Model file for the job. Use its own axes, mm. A direction names the side the tool comes from. Coordinates: 2 decimals unless noted, no trailing zeros. Loops run counter-clockwise (first coordinate to the right, second up) from the corner with the lowest first, then second, coordinate; pieces in that order, holes last. Notation, with made-up numbers: (-12.75, 88.5) -> (28.25, 88.5) arc R33 ccw to (28.25, 120.5) -> close; hole circle Ø5 at (75, 76.25). An arc over 180 degrees is marked (long way). Use one line per item in the form item = value.
```python
from build123d import *

# Parameters (mm, degrees)
SKETCH_1_R          = 24.5
SKETCH_1_R_2        = 2.1
EXTRUDE_1_DEPTH     = 2
CUT_EXTRUDE_1_DEPTH = 10


with BuildPart() as part:
    # 草图1 → 凸台-拉伸1 (new body)
    with BuildSketch(Plane.XY):
        with BuildLine():
            Line((-50, 15), (-50, -15))
            ThreePointArc((-50, -15), (-49.077002077, -17.894486839), (-46.648778375, -19.720331542))
            Line((-46.648778375, -19.720331542), (-11.211692948, -32.098254489))
            ThreePointArc((-11.211692948, -32.098254489), (0, -34), (11.211692948, -32.098254489))
            Line((11.211692948, -32.098254489), (46.648778375, -19.720331542))
            ThreePointArc((46.648778375, -19.720331542), (49.077002077, -17.894486839), (50, -15))
            Line((50, -15), (50, 15))
            ThreePointArc((50, 15), (49.077002077, 17.894486839), (46.648778375, 19.720331542))
            Line((46.648778375, 19.720331542), (11.211692948, 32.098254489))
            ThreePointArc((11.211692948, 32.098254489), (0, 34), (-11.211692948, 32.098254489))
            Line((-11.211692948, 32.098254489), (-46.648778375, 19.720331542))
            ThreePointArc((-46.648778375, 19.720331542), (-49.077002077, 17.894486839), (-50, 15))
        make_face()
        Circle(SKETCH_1_R, mode=Mode.SUBTRACT)
        with Locations((0, 29)):
            Circle(SKETCH_1_R_2, mode=Mode.SUBTRACT)
        with Locations((25.11473671, 14.5)):
            Circle(SKETCH_1_R_2, mode=Mode.SUBTRACT)
        with Locations((25.11473671, -14.5)):
            Circle(SKETCH_1_R_2, mode=Mode.SUBTRACT)
        with Locations((0, -29)):
            Circle(SKETCH_1_R_2, mode=Mode.SUBTRACT)
        with Locations((-25.11473671, -14.5)):
            Circle(SKETCH_1_R_2, mode=Mode.SUBTRACT)
        with Locations((-25.11473671, 14.5)):
            Circle(SKETCH_1_R_2, mode=Mode.SUBTRACT)
        with Locations((-45, 15)):
            Circle(SKETCH_1_R_2, mode=Mode.SUBTRACT)
        with Locations((-45, -15)):
            Circle(SKETCH_1_R_2, mode=Mode.SUBTRACT)
        with Locations((45, -15)):
            Circle(SKETCH_1_R_2, mode=Mode.SUBTRACT)
        with Locations((45, 15)):
            Circle(SKETCH_1_R_2, mode=Mode.SUBTRACT)
    extrude(amount=EXTRUDE_1_DEPTH)

    # 草图2 → 切除-拉伸1 (cut)
    with BuildSketch(Plane.XY.offset(2)):
        with BuildLine():
            Line((-43, 11), (-31, 11))
            ThreePointArc((-31, 11), (-29.585786438, 10.414213562), (-29, 9))
            Line((-29, 9), (-29, -9))
            ThreePointArc((-29, -9), (-29.585786438, -10.414213562), (-31, -11))
            Line((-31, -11), (-43, -11))
            ThreePointArc((-43, -11), (-44.414213562, -10.414213562), (-45, -9))
            Line((-45, -9), (-45, 9))
            ThreePointArc((-45, 9), (-44.414213562, 10.414213562), (-43, 11))
        make_face()
        with BuildLine():
            Line((31, 11), (43, 11))
            ThreePointArc((43, 11), (44.414213562, 10.414213562), (45, 9))
            Line((45, 9), (45, -9))
            ThreePointArc((45, -9), (44.414213562, -10.414213562), (43, -11))
            Line((43, -11), (31, -11))
            ThreePointArc((31, -11), (29.585786438, -10.414213562), (29, -9))
            Line((29, -9), (29, 9))
            ThreePointArc((29, 9), (29.585786438, 10.414213562), (31, 11))
        make_face()
    extrude(amount=-CUT_EXTRUDE_1_DEPTH, mode=Mode.SUBTRACT)


solid = part.part
```
Q1. Mould opens along Y. For faces 1 (the face through (29.6, -10.43, 1.01)), 2 (the face through (-15, -20, 0)), 3 (the face through (49, 18, 1)), 4 (the face through (0, -34, 1)) say: released by +Y, released by -Y, zero draft, split by the parting line, or undercut.
Result:
face_1 = undercut
face_2 = zero draft
face_3 = released by +Y
face_4 = released by -Y
Q2. Pin check, flat tips, straight feed: pin 1 Ø0.6 at (x, z) = (35, 1.5) entering from -Y; pin 2 Ø6 at (x, y) = (-5.5, -22) entering from +Z; pin 3 Ø0.6 at (x, z) = (39, 1.5) entering from +Y; pin 4 Ø1 at (x, z) = (-16.5, 0.5) entering from -Y. Stop position of each tip, or through.
Result:
pin_1 = -23.89
pin_2 = 2
pin_3 = 22.5
pin_4 = -30.43
Q3. Which spindle directions (+Z, -Z, +X, -X, +Y, -Y) get a long thin tool onto all of the face, cutting with end or side? Do faces 5 (the face through (-44.43, 10.4, 1.01)), 6 (the face through (28.682, -25.996, 0.986)). Say none if no direction does.
Result:
face_5 = +Z, -Z
face_6 = +Z, -Z, +X, -Y
Q4. Band-saw the part on A-A, the plane y = 0. Write the cut outline in (x, z).
Result:
outline = (-50, 0) -> (-45, 0) -> (-45, 2) -> (-50, 2) -> close; (-29, 0) -> (-24.5, 0) -> (-24.5, 2) -> (-29, 2) -> close; (24.5, 0) -> (29, 0) -> (29, 2) -> (24.5, 2) -> close; (45, 0) -> (50, 0) -> (50, 2) -> (45, 2) -> close
Q5. Wall check: line 1 along Y through (x, z) = (0, 0.9); line 2 along X through (y, z) = (1.5, 0.55); line 3 along Y through (x, z) = (-44.5, 1.65). Give the ranges that are in metal, low to high.
Result:
line_1 = -34 to -31.1, -26.9 to -24.5, 24.5 to 26.9, 31.1 to 34
line_2 = -50 to -45, -29 to -24.45, 24.45 to 29, 45 to 50
line_3 = -20.47 to -17.04, -12.96 to -10.32, 10.32 to 12.96, 17.04 to 20.47
Q6. Band-saw the part on D-D, the plane x = 17.5. Write the cut outline in (y, z).
Result:
outline = (-29.9, 0) -> (-17.15, 0) -> (-17.15, 2) -> (-29.9, 2) -> close; (17.15, 0) -> (29.9, 0) -> (29.9, 2) -> (17.15, 2) -> close
Q7. Band-saw the part on B-B, the plane x = 0. Write the cut outline in (y, z), and give its area (3 significant figures).
Result:
outline = (-34, 0) -> (-31.1, 0) -> (-31.1, 2) -> (-34, 2) -> close; (-26.9, 0) -> (-24.5, 0) -> (-24.5, 2) -> (-26.9, 2) -> close; (24.5, 0) -> (26.9, 0) -> (26.9, 2) -> (24.5, 2) -> close; (31.1, 0) -> (34, 0) -> (34, 2) -> (31.1, 2) -> close
area = 21.2 mm2
Q8. Band-saw the part on C-C, the plane y = 29. Write the cut outline in (x, z).
Result:
outline = (-20.08, 0) -> (-2.1, 0) -> (-2.1, 2) -> (-20.08, 2) -> close; (2.1, 0) -> (20.08, 0) -> (20.08, 2) -> (2.1, 2) -> close
